Source: CAD feature listing. Evaluate the final solid. Frame: model axes, mm. A direction names the side the tool comes from. Coordinates: 2 decimals unless noted, no trailing zeros. Write each loop counter-clockwise with the first axis right and the second up, starting at its lowest first coordinate (ties: lowest second). Pieces come first, ordered by that corner, then holes. Notation, with made-up numbers: (-15, -36) -> (-3, -36) arc R30 ccw to (-3, -6) -> close; hole circle Ø10 at (20.25, 37). An arc over 180 degrees is marked (long way). One line per item, written item: value. Start each with the question number.
1. Section query B-B, the plane z = 8. State how many separate pieces and enclosed holes the cut face has, and give its area (3 significant figures).
2. Mould query, pull axis X, two halves, no side actions, for faces 4 (the flat face through (-1, -52, 6)), 5 (the flat face through (148, -185.5, 6)), 6 (the flat face through (-200, -91, 6)). Classes: released by +X, released by -X, zero draft, split by the parting line, or undercut.
3. Section query C-C, the plane x = 26. Output: boundary loops of the cut face in (y, z), and give its area (3 significant figures).
4. Access query for faces 1 (the flat face through (155, -150.25, 6)), 2 (the flat face through (-3, -50, 12)), 3 (the flat face through (98, -123, 6)). Directions: +Z, -Z, +X, -X, +Y, -Y. A direction counts if a zero-diameter tool reaches every point of the face in a straight line with its end or side. Return the directions, or none.
5. Line query: line 1 (Y direction, x = 176, z = 4); line 2 (X direction, y = -165, z = 9.75); line 3 (X direction, y = -56.5, z = 5.5). Output: solid intervals per line, ascending.
6. First-contact query: P1, Ø3, axis at x = 96, z = 1.5, coming from the -Y side. Flat tip, straight axial feed; report the tip coordinate or a pass-through.
7. Section query A-A, the plane y = -99. Output: boundary loops of the cut face in (x, z), and give its area (3 significant figures).
from build123d import *

# Parameters (mm, degrees)
F0_W     = 60
F0_H     = 8
F1_DEPTH = 12
F2_R     = 1
F3_R     = 3.99999


# Not quite as in the source:
# - a fillet or chamfer is up to 0.001 mm smaller than in the source, because OpenCascade refuses the exact size


with BuildPart() as f1:
    # F0 (on Top) → F1 (new body)
    with BuildSketch(Plane.XY):
        with BuildLine():
            Line((200, 0), (-200, 0))
            Line((-200, 0), (-200, -185.5))
            Line((-200, -185.5), (-98, -185.5))
            Line((-98, -185.5), (-98, -61.8994949366))
            ThreePointArc((-98, -61.8994949366), (-98, -52), (-88.1005050634, -52))
            Line((-88.1005050634, -52), (88.1005050634, -52))
            ThreePointArc((88.1005050634, -52), (98, -52), (98, -61.8994949366))
            Line((98, -61.8994949366), (98, -185.5))
            Line((98, -185.5), (200, -185.5))
            Line((200, -185.5), (200, 0))
        make_face()
        with Locations((155, -154.25)):
            Rectangle(F0_W, F0_H, mode=Mode.SUBTRACT)
        with Locations((155, -79.25)):
            Rectangle(F0_W, F0_H, mode=Mode.SUBTRACT)
    extrude(amount=F1_DEPTH)

    # F2
    f2_edges = [f1.edges().sort_by_distance(p)[0] for p in [
        (-98, -185.5, 6),
        (-98, -61.899495, 6),
        (-88.100505, -52, 6),
        (88.100505, -52, 6),
        (98, -61.899495, 6),
        (98, -185.5, 6),
        (200, -185.5, 6),
        (200, 0, 6),
        (-200, 0, 6),
        (-200, -185.5, 6),
    ]]
    fillet(f2_edges, radius=F2_R)

    # F3 (radius 4 in the source; OpenCascade refuses exactly that, so slightly less here)
    f3_edges = [f1.edges().sort_by_distance(p)[0] for p in [
        (125, -158.25, 6),
        (125, -150.25, 6),
        (185, -158.25, 6),
        (185, -150.25, 6),
        (125, -83.25, 6),
        (125, -75.25, 6),
        (185, -83.25, 6),
        (185, -75.25, 6),
    ]]
    fillet(f3_edges, radius=F3_R)


solid = f1.part
Computed values:
1. separate pieces: 1
1. enclosed holes: 2
1. area: 47,000 mm²
2. face 4: undercut
2. face 5: zero draft
2. face 6: released by -X
3. outline: (-52, 0) -> (0, 0) -> (0, 12) -> (-52, 12) -> close
3. area: 624 mm²
4. face 1: +Z, -Z
4. face 2: +Z, +X, -X, +Y, -Y
4. face 3: +Z, -Z, -Y
5. line 1: y = -185.5 to -158.25, -150.25 to -83.25, -75.25 to 0
5. line 2: x = -200 to -98, 98 to 200
5. line 3: x = -200 to -100.04, 100.04 to 200
6. P1: stops at y = -51.55
7. outline: (-200, 0) -> (-98, 0) -> (-98, 12) -> (-200, 12) -> close; (98, 0) -> (200, 0) -> (200, 12) -> (98, 12) -> close
7. area: 2,450 mm²
